Could you check a few things on this model? Use its own coordinates, in mm. Face numbers are marked on the shaded views. A direction names the side the tool comes from. Give positions to 0.01 mm unless a question says otherwise; leave off trailing zeros. Order: outer loops, then holes, each group sorted by start corner. A loop starts at its lowest first (then second) coordinate and runs counter-clockwise, first axis right, second up. Notation, with made-up numbers: (56, 76.5) -> (63, 76.5) arc R23 ccw to (63, 91.5) -> close; hole circle Ø6 at (19, 53). An arc over 180 degrees is marked (long way). Write each question's results on one line, items separated by ' | '.
```python
from build123d import *

# Parameters (mm, degrees)
SKETCH_1_W             = 175
SKETCH_1_H             = 65
EXTRUDE_1_DEPTH        = 1.5
SKETCH_3_W             = 175
SKETCH_3_H             = 65
SKETCH_3_W_2           = 171
SKETCH_3_H_2           = 61
EXTRUDE_2_DEPTH        = 20
SKETCH_4_W             = 40
SKETCH_4_H             = 20
CUT_EXTRUDE_1_DEPTH    = 2
SKETCH_6_R             = 2.25
CUT_EXTRUDE_2_DEPTH    = 2
SKETCH_9_W             = 2
SKETCH_9_H             = 61
EXTRUDE_4_DEPTH        = 20
SKETCH_12_W            = 4
SKETCH_12_H            = 10
CUT_EXTRUDE_4_DEPTH    = 2
CHAMFER_1_SIZE         = 3
CHAMFER_2_SIZE         = 3
CHAMFER_3_SIZE         = 1.5
SKETCH_13_R            = 4.5
CUT_EXTRUDE_5_DEPTH    = 71
PATTERN_LINEAR_1_COUNT = 7
PATTERN_LINEAR_1_PITCH = 18
SKETCH_14_W            = 2
SKETCH_14_H            = 61
EXTRUDE_5_DEPTH        = 20
CHAMFER_4_SIZE         = 3
CHAMFER_5_SIZE         = 3
SKETCH_15_R            = 4.5
CUT_EXTRUDE_6_DEPTH    = 71
PATTERN_LINEAR_2_COUNT = 4
PATTERN_LINEAR_2_PITCH = 15
CUT_EXTRUDE_7_DEPTH    = 4
SKETCH_18_W            = 27
SKETCH_18_H            = 4
CUT_EXTRUDE_8_DEPTH    = 5
CUT_EXTRUDE_9_DEPTH    = 10


# Some blends are built 0.0001 mm under size
with BuildPart() as part:
    # Эскиз1 → Бобышка-Вытянуть1 (new body)
    with BuildSketch(Plane(origin=(0, 0, 0), x_dir=(1, 0, 0), z_dir=(0, 1, 0))):
        Rectangle(SKETCH_1_W, SKETCH_1_H)
    extrude(amount=EXTRUDE_1_DEPTH)

    # Эскиз3 → Бобышка-Вытянуть2 (add)
    with BuildSketch(Plane(origin=(0, 1.5, 0), x_dir=(1, 0, 0), z_dir=(0, 1, 0))):
        Rectangle(SKETCH_3_W, SKETCH_3_H)
        Rectangle(SKETCH_3_W_2, SKETCH_3_H_2, mode=Mode.SUBTRACT)
    extrude(amount=EXTRUDE_2_DEPTH)

    # Эскиз4 → Вырез-Вытянуть1 (cut)
    with BuildSketch(Plane(origin=(87.5, 0, 0), x_dir=(0, 0, -1), z_dir=(1, 0, 0))):
        with Locations((0, 11.5)):
            Rectangle(SKETCH_4_W, SKETCH_4_H)
    extrude(amount=-CUT_EXTRUDE_1_DEPTH, mode=Mode.SUBTRACT)

    # Эскиз6 → Вырез-Вытянуть2 (cut)
    with BuildSketch(Plane(origin=(87.5, 0, 0), x_dir=(0, 0, -1), z_dir=(1, 0, 0))):
        with Locations((-24, 7.25)):
            Circle(SKETCH_6_R)
        with BuildLine():
            Line((-21.75, 16.918419021), (-21.75, 13.918419021))
            ThreePointArc((-21.75, 13.918419021), (-24, 11.668419021), (-26.25, 13.918419021))
            Line((-26.25, 13.918419021), (-26.25, 16.918419021))
            ThreePointArc((-26.25, 16.918419021), (-24, 19.168419021), (-21.75, 16.918419021))
        make_face()
    cut_extrude_2 = extrude(amount=-CUT_EXTRUDE_2_DEPTH, mode=Mode.SUBTRACT)

    # Зеркальное отражение2: Вырез-Вытянуть2 across plane
    add(cut_extrude_2.mirror(Plane(origin=(0, 0, 0), x_dir=(1, 0, 0), z_dir=(0, 0, -1))), mode=Mode.SUBTRACT)

    # Эскиз9 → Бобышка-Вытянуть4 (add)
    with BuildSketch(Plane(origin=(0, 1.5, 0), x_dir=(1, 0, 0), z_dir=(0, 1, 0))):
        with Locations((50.5, 0)):
            Rectangle(SKETCH_9_W, SKETCH_9_H)
    extrude(amount=EXTRUDE_4_DEPTH)

    # Эскиз12 → Вырез-Вытянуть4 (cut)
    with BuildSketch(Plane(origin=(51.5, 0, 0), x_dir=(0, 0, -1), z_dir=(1, 0, 0))):
        with Locations((-25.5, 11.5)):
            Rectangle(SKETCH_12_W, SKETCH_12_H)
    extrude(amount=-CUT_EXTRUDE_4_DEPTH, mode=Mode.SUBTRACT)

    # Фаска1
    chamfer_1_edges = [part.edges().sort_by_distance(p)[0] for p in [
        (-85.5, 11.5, -30.5),
        (-85.5, 11.5, 30.5),
        (49.5, 11.5, -30.5),
        (49.5, 11.5, 30.5),
    ]]
    chamfer(chamfer_1_edges, length=CHAMFER_1_SIZE - 0.0001)  # a hair under: the kernel refuses the full size

    # Фаска2
    chamfer_2_edges = [part.edges().sort_by_distance(p)[0] for p in [
        (51.5, 11.5, 30.5),
        (51.5, 11.5, -30.5),
    ]]
    chamfer(chamfer_2_edges, length=CHAMFER_2_SIZE - 0.0001)  # a hair under: the kernel refuses the full size

    # Фаска3
    chamfer_3_edges = [part.edges().sort_by_distance(p)[0] for p in [
        (85.5, 11.5, 30.5),
        (85.5, 11.5, -30.5),
    ]]
    chamfer(chamfer_3_edges, length=CHAMFER_3_SIZE)

    # Эскиз13 → Вырез-Вытянуть5 (cut)
    with BuildSketch(Plane(origin=(0, 0, -32.5), x_dir=(-1, 0, 0), z_dir=(0, 0, -1))):
        with Locations((-39.5, 10.75)):
            Circle(SKETCH_13_R)
    cut_extrude_5 = extrude(amount=-CUT_EXTRUDE_5_DEPTH, mode=Mode.SUBTRACT)

    # Линейный массив1: Вырез-Вытянуть5 ×7
    with Locations(*[(-i * PATTERN_LINEAR_1_PITCH, 0, 0) for i in range(1, PATTERN_LINEAR_1_COUNT)]):
        add(cut_extrude_5, mode=Mode.SUBTRACT)

    # Эскиз14 → Бобышка-Вытянуть5 (add)
    with BuildSketch(Plane(origin=(0, 1.5, 0), x_dir=(1, 0, 0), z_dir=(0, 1, 0))):
        with Locations((-24.5, 0)):
            Rectangle(SKETCH_14_W, SKETCH_14_H)
    extrude(amount=EXTRUDE_5_DEPTH)

    # Фаска4
    # the kernel refuses this chamfer: 3 mm, written as the material it adds along each edge
    with BuildSketch(Plane(origin=(-25.5, 1.5, -30.5), x_dir=(-0.9996219169112968, 0, -0.027495876610586733), z_dir=(0, 1, 0))) as chamfer_4_piece_1_section:
        Polygon((CHAMFER_4_SIZE * 0.999621916911, CHAMFER_4_SIZE * 0.0274958766106), (-CHAMFER_4_SIZE * 0.0274958766106, CHAMFER_4_SIZE * 0.999621916911), (0, 0), align=None)
    chamfer_4_piece_1 = extrude(amount=20, mode=Mode.PRIVATE)
    chamfer_4_piece_1 = chamfer_4_piece_1 - Plane(origin=(-32.5, 10.75, -29.506003932), x_dir=(-1, 0, 0), z_dir=(0, 0, -1)) * Cylinder(4.5, 52, mode=Mode.PRIVATE)
    add(chamfer_4_piece_1)
    with BuildSketch(Plane(origin=(-25.5, 1.5, 30.5), x_dir=(-0.9996219169112968, 0, 0.0274958766105868), z_dir=(0, 1, 0))) as chamfer_4_piece_2_section:
        Polygon((CHAMFER_4_SIZE * 0.999621916911, -CHAMFER_4_SIZE * 0.0274958766106), (-CHAMFER_4_SIZE * 0.0274958766106, -CHAMFER_4_SIZE * 0.999621916911), (0, 0), align=None)
    chamfer_4_piece_2 = extrude(amount=20, mode=Mode.PRIVATE)
    chamfer_4_piece_2 = chamfer_4_piece_2 - Plane(origin=(-32.5, 10.75, 29.506003932), x_dir=(-1, 0, 0), z_dir=(0, 0, -1)) * Cylinder(4.5, 52, mode=Mode.PRIVATE)
    add(chamfer_4_piece_2)

    # Фаска5
    chamfer_5_edges = [part.edges().sort_by_distance(p)[0] for p in [
        (-23.5, 11.5, 30.5),
        (-23.5, 11.5, -30.5),
    ]]
    chamfer(chamfer_5_edges, length=CHAMFER_5_SIZE)

    # Эскиз15 → Вырез-Вытянуть6 (cut)
    with BuildSketch(Plane(origin=(-23.5, 0, 0), x_dir=(0, 0, -1), z_dir=(1, 0, 0))):
        with Locations((-22.5, 11.5)):
            Circle(SKETCH_15_R)
    cut_extrude_6 = extrude(amount=-CUT_EXTRUDE_6_DEPTH, mode=Mode.SUBTRACT)

    # Линейный массив2: Вырез-Вытянуть6 ×4
    with Locations(*[(0, 0, -i * PATTERN_LINEAR_2_PITCH) for i in range(1, PATTERN_LINEAR_2_COUNT)]):
        add(cut_extrude_6, mode=Mode.SUBTRACT)

    # Эскиз16 → Вырез-Вытянуть7 (cut)
    with BuildSketch(Plane(origin=(0, 1.5, 0), x_dir=(1, 0, 0), z_dir=(0, 1, 0))):
        with BuildLine():
            Line((6.8, 14.5), (11.8, 14.5))
            ThreePointArc((11.8, 14.5), (13.3, 13), (11.8, 11.5))
            Line((11.8, 11.5), (6.8, 11.5))
            ThreePointArc((6.8, 11.5), (5.3, 13), (6.8, 14.5))
        make_face()
        with BuildLine():
            Line((39.5, 14.5), (44.5, 14.5))
            ThreePointArc((44.5, 14.5), (46, 13), (44.5, 11.5))
            Line((44.5, 11.5), (39.5, 11.5))
            ThreePointArc((39.5, 11.5), (38, 13), (39.5, 14.5))
        make_face()
    extrude(amount=-CUT_EXTRUDE_7_DEPTH, mode=Mode.SUBTRACT)

    # Эскиз18 → Вырез-Вытянуть8 (cut)
    with BuildSketch(Plane(origin=(0, 1.5, 0), x_dir=(1, 0, 0), z_dir=(0, 1, 0))):
        with Locations((-57, 22)):
            Rectangle(SKETCH_18_W, SKETCH_18_H)
        with Locations((-54.553283303, -22)):
            Rectangle(SKETCH_18_W, SKETCH_18_H)
    extrude(amount=-CUT_EXTRUDE_8_DEPTH, mode=Mode.SUBTRACT)

    # Эскиз19 → Вырез-Вытянуть9 (cut)
    with BuildSketch(Plane(origin=(0, 1.5, 0), x_dir=(1, 0, 0), z_dir=(0, 1, 0))):
        with BuildLine():
            Line((83.75, 21.5), (83.75, 19.5))
            ThreePointArc((83.75, 19.5), (82.5, 18.25), (81.25, 19.5))
            Line((81.25, 19.5), (81.25, 21.5))
            ThreePointArc((81.25, 21.5), (82.5, 22.75), (83.75, 21.5))
        make_face()
        with BuildLine():
            Line((83.75, -18.5), (83.75, -20.5))
            ThreePointArc((83.75, -20.5), (82.5, -21.75), (81.25, -20.5))
            Line((81.25, -20.5), (81.25, -18.5))
            ThreePointArc((81.25, -18.5), (82.5, -17.25), (83.75, -18.5))
        make_face()
        with BuildLine():
            Line((-81.25, 19.5), (-81.25, 17.5))
            ThreePointArc((-81.25, 17.5), (-82.5, 16.25), (-83.75, 17.5))
            Line((-83.75, 17.5), (-83.75, 19.5))
            ThreePointArc((-83.75, 19.5), (-82.5, 20.75), (-81.25, 19.5))
        make_face()
        with BuildLine():
            Line((-81.25, -18.5), (-81.25, -20.5))
            ThreePointArc((-81.25, -20.5), (-82.5, -21.75), (-83.75, -20.5))
            Line((-83.75, -20.5), (-83.75, -18.5))
            ThreePointArc((-83.75, -18.5), (-82.5, -17.25), (-81.25, -18.5))
        make_face()
    extrude(amount=-CUT_EXTRUDE_9_DEPTH, mode=Mode.SUBTRACT)


solid = part.part
```
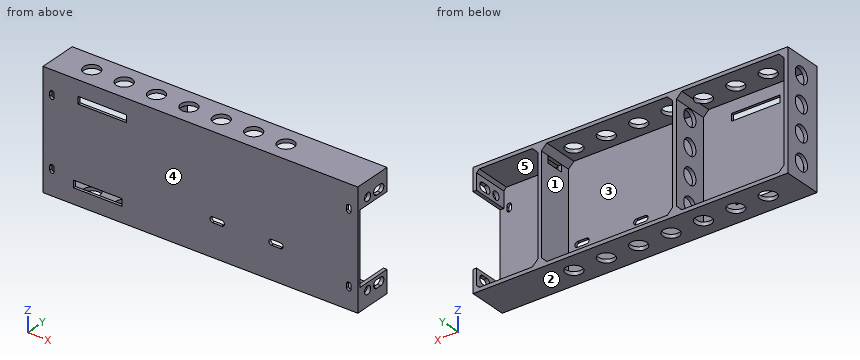
Q1. Suppose I cut it at A-A on x = -14.5. Please give me the cut outline in (y, z), and give its area (4 significant figures).
Here are the results:
outline: (0, -32.5) -> (6.25, -32.5) -> (6.25, -30.5) -> (1.5, -30.5) -> (1.5, 30.5) -> (6.25, 30.5) -> (6.25, 32.5) -> (0, 32.5) -> close; (15.25, -32.5) -> (21.5, -32.5) -> (21.5, -30.5) -> (15.25, -30.5) -> close; (15.25, 30.5) -> (21.5, 30.5) -> (21.5, 32.5) -> (15.25, 32.5) -> close | area: 141.5 mm²
Q2. Suppose I cut it at B-B on z = 1. Please give me the cut outline in (x, y).
Here are the results:
outline: (-87.5, 0) -> (87.5, 0) -> (87.5, 1.5) -> (51.5, 1.5) -> (51.5, 21.5) -> (49.5, 21.5) -> (49.5, 1.5) -> (-23.5, 1.5) -> (-23.5, 21.5) -> (-25.5, 21.5) -> (-25.5, 1.5) -> (-85.5, 1.5) -> (-85.5, 21.5) -> (-87.5, 21.5) -> close
Q3. For the marked faces 4 and 5, which set-ups out of +Z, -Z, +X, -X, +Y, -Y let a thin tool reach every point of the face, with its end or its side?
Here are the results:
face 4: +Z, -Z, +X, -X, -Y | face 5: +Y
Q4. I need wall thicknesses on line 1 along X through (y, z) = (12.75, -13); line 2 along Z through (x, y) = (-67, 20.75); line 3 along Z through (x, y) = (-65.5, 1.25). Which ranges of each line are inside material? Lowest first, please.
Here are the results:
line 1: x = -87.5 to -85.5, -25.5 to -23.5, 49.5 to 51.5 | line 2: z = -32.5 to -30.5, 30.5 to 32.5 | line 3: z = -32.5 to -24, -20 to 20, 24 to 32.5
Q5. I'm going to push flat-ended pins straight in: pin 1 Ø12 at (x, z) = (6, 3.5) entering from +Y; pin 2 Ø10 at (y, z) = (18, 8.5) entering from +X. Where does each tip first touch, or does it pass through?
Here are the results:
pin 1: stops at y = 1.5 | pin 2: stops at x = 51.5
Q6. Thinking about a two-plate mould opening in X: for the marked faces 1, 2 and 3, which applies, +X half, -X half, draft (parallel to the pull), parting line (faces both ways), or undercut?
Here are the results:
face 1: undercut | face 2: draft | face 3: undercut
Q7. Suppose I cut it at C-C on x = 32.5. Please give me the cut outline in (y, z), and give its area (4 significant figures).
Here are the results:
outline: (0, -32.5) -> (21.5, -32.5) -> (21.5, -30.5) -> (1.5, -30.5) -> (1.5, 30.5) -> (21.5, 30.5) -> (21.5, 32.5) -> (0, 32.5) -> close | area: 177.5 mm²
